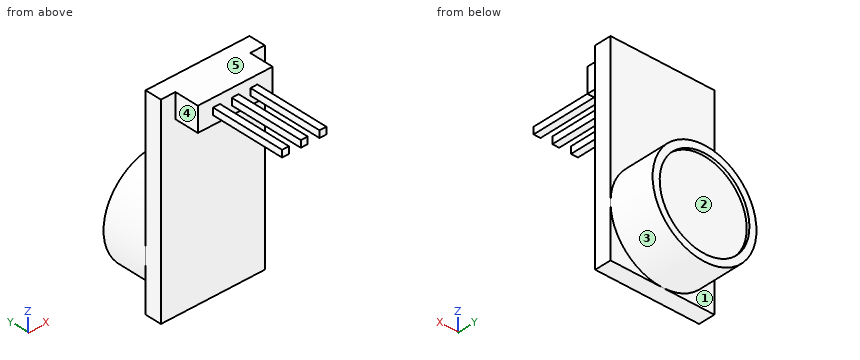
from build123d import *

# Parameters (mm, degrees)
SKETCH1_W           = 10.7
SKETCH1_H           = 20.6
BOSS_EXTRUDE1_DEPTH = 0.85
SKETCH2_R           = 5.35
BOSS_EXTRUDE2_DEPTH = 6.4
SKETCH3_W           = 7.7
SKETCH3_H           = 2.5
BOSS_EXTRUDE3_DEPTH = 2.5
SKETCH4_W           = 0.707106782
SKETCH4_H           = 0.707106782
BOSS_EXTRUDE4_DEPTH = 7.7
SKETCH5_R           = 4.620940101
CUT_EXTRUDE1_DEPTH  = 0.3


with BuildPart() as part:
    # Sketch1 → Boss-Extrude1 (new, symmetric)
    with BuildSketch(Plane(origin=(0, 0, 0), x_dir=(1, 0, 0), z_dir=(0, 1, 0))):
        Rectangle(SKETCH1_W, SKETCH1_H)
    extrude(amount=BOSS_EXTRUDE1_DEPTH, both=True)

    # Sketch2 → Boss-Extrude2 (add)
    with BuildSketch(Plane.XZ.offset(0.85)):
        with Locations(Location((0, -4.95, 0), (0, 0, 270))):
            Circle(SKETCH2_R)
    extrude(amount=-BOSS_EXTRUDE2_DEPTH)

    # Sketch3 → Boss-Extrude3 (add)
    with BuildSketch(Plane.XZ.offset(0.85)):
        with Locations((0, 9.05)):
            Rectangle(SKETCH3_W, SKETCH3_H)
    extrude(amount=BOSS_EXTRUDE3_DEPTH)

    # Sketch4 → Boss-Extrude4 (add)
    with BuildSketch(Plane.XZ.offset(3.35)):
        with Locations((-1.925, 9.05)):
            Rectangle(SKETCH4_W, SKETCH4_H)
        with Locations((0, 9.05)):
            Rectangle(SKETCH4_W, SKETCH4_H)
        with Locations((1.925, 9.05)):
            Rectangle(SKETCH4_W, SKETCH4_H)
    extrude(amount=BOSS_EXTRUDE4_DEPTH)

    # Sketch5 → Cut-Extrude1 (cut)
    with BuildSketch(Plane(origin=(0, 5.55, 0), x_dir=(1, 0, 0), z_dir=(0, 1, 0))):
        with Locations(Location((0, 4.95, 0), (0, 0, 270))):
            Circle(SKETCH5_R)
    extrude(amount=-CUT_EXTRUDE1_DEPTH, mode=Mode.SUBTRACT)


solid = part.part
Read the model definition and answer for the solid it produces. Units are mm, in the model's axes. Face numbers are marked on the shaded views. A direction names the side the tool comes from. Give positions to 0.01 mm unless a question says otherwise; leave off trailing zeros. Write each loop counter-clockwise with the first axis right and the second up, starting at its lowest first coordinate (ties: lowest second). Pieces come first, ordered by that corner, then holes. Notation, with made-up numbers: (-9.75, -25) - (-4.75, -25) arc R17 cw to (-4.75, 5) - close; hole circle Ø9 at (75.5, -29.75). An arc over 180 degrees is marked (long way). Answer in a Markdown table with one row per item. Add a question column.
Item 1: Determine the mould class of the marked faces 1, 2 and 3 for opening direction Z: pulls with the +Z half, pulls with the -Z half, needs draft (parallel to the pull), parting line crosses it, or undercut.
Item 2: A tool of negligible diameter and unlimited length cuts with its end or side. For the marked faces 4 and 5, from which of +Z, -Z, +X, -X, +Y, -Y can it reach the whole face along a straight path? Write none if from no direction.
Item 3: Section D-D, the plane z = -1 is taken. Write down the section's boundary in (x, y).
Item 4: Find the intervals of material crossed by L1, parallel to X at y = 5.45, z = -4.95; L2, parallel to Y at x = 1.5, z = -3.25; L3, parallel to Y at x = -0.5, z = 0, in increasing order.
Item 5: Flat-ended cylindrical pins translate along their axes: P1, Ø0.6, axis at x = 2, y = -5.5, coming from the +Z side; P2, Ø0.8, axis at x = 0, y = -2.5, coming from the -Z side; P3, Ø6, axis at x = 2, z = 5.5, coming from the -Y side. Find the tip coordinate at first contact, or state that the pin passes through.
Item 6: Section A-A, the plane z = -8.25 is taken. Write down the section's boundary in (x, y), and give its area (3 significant figures).
Item 7: Section C-C, the plane x = -2 is taken. Write down the section's boundary in (y, z), and give its area (3 significant figures).
Item 8: Section B-B, the plane y = 4 is taken. Write down the section's boundary in (x, z).
Recorded:
| question | item | result |
|---|---|---|
| 1 | face 1 | needs draft |
| 1 | face 2 | undercut |
| 1 | face 3 | parting line crosses it |
| 2 | face 4 | +Z, -Z, -X, -Y |
| 2 | face 5 | +Z, +X, -X, +Y, -Y |
| 3 | outline | (-5.35, -0.85) - (5.35, -0.85) - (5.35, 0.85) - (3.61, 0.85) - (3.61, 5.55) - (2.4, 5.55) - (2.4, 5.25) - (-2.4, 5.25) - (-2.4, 5.55) - (-3.61, 5.55) - (-3.61, 0.85) - (-5.35, 0.85) - close |
| 4 | L1 | x = -5.35 to -4.62, 4.62 to 5.35 |
| 4 | L2 | y = -0.85 to 5.25 |
| 4 | L3 | y = -0.85 to 5.55 |
| 5 | P1 | stops at z = 9.4 |
| 5 | P2 | stops at z = 7.8 |
| 5 | P3 | stops at y = -3.35 |
| 6 | outline | (-5.35, -0.85) - (5.35, -0.85) - (5.35, 0.85) - (4.21, 0.85) - (4.21, 5.55) - (3.23, 5.55) - (3.23, 5.25) - (-3.23, 5.25) - (-3.23, 5.55) - (-4.21, 5.55) - (-4.21, 0.85) - (-5.35, 0.85) - close |
| 6 | area | 55.8 mm2 |
| 7 | outline | (-11.05, 8.7) - (-3.35, 8.7) - (-3.35, 7.8) - (-0.85, 7.8) - (-0.85, -10.3) - (0.85, -10.3) - (0.85, -9.91) - (5.55, -9.91) - (5.55, -9.12) - (5.25, -9.12) - (5.25, -0.78) - (5.55, -0.78) - (5.55, 0.01) - (0.85, 0.01) - (0.85, 10.3) - (-3.35, 10.3) - (-3.35, 9.4) - (-11.05, 9.4) - close |
| 7 | area | 90.9 mm2 |
| 8 | outline | circle Ø10.7 at (0, -4.95) |
